For this review, take the finished solid that the model builds, in its own axes (mm). A direction names the side the tool comes from. Round coordinates to 2 decimals unless told otherwise and drop trailing zeros. Write each loop counter-clockwise with the first axis right and the second up, starting at its lowest first coordinate (ties: lowest second). Pieces come first, ordered by that corner, then holes. Notation, with made-up numbers: M 14,-7 L 54,-7 A24 cw 54,31 Z; hole C -28.75,-26.75 d2. An arc over 180 degrees is marked long. One line per question, with ' | ' between items.
```python
from build123d import *

# Parameters (mm, degrees)
BOSS_EXTRUDE1_DEPTH = 50.8
CUT_EXTRUDE2_REACH  = 8.35
SKETCH4_R           = 2.54
CUT_EXTRUDE1_REACH  = 8.35
SKETCH3_R           = 2.54
SKETCH3_R_2         = 14.224
CUT_EXTRUDE3_DEPTH  = 3.81


with BuildPart() as part:
    # Sketch2 → Boss-Extrude1 (new body)
    with BuildSketch(Plane(origin=(0, 0, 0), x_dir=(1, 0, 0), z_dir=(0, 1, 0))):
        Polygon((0, 58.372586566), (0, 0), (48.980415858, 0), (43.6521332, 6.35), (6.35, 6.35), (6.35, 50.804951253), align=None)
    extrude(amount=BOSS_EXTRUDE1_DEPTH)

    # Sketch4 → Cut-Extrude2 (cut, up to next)
    with BuildSketch(Plane(origin=(0, 0, -6.35), x_dir=(-1, 0, 0), z_dir=(0, 0, -1)), mode=Mode.PRIVATE) as cut_extrude2_sk1:
        with Locations((-37.7010666, 36.83)):
            Circle(SKETCH4_R)
    cut_extrude2_tool1 = extrude(cut_extrude2_sk1.sketch, amount=-CUT_EXTRUDE2_REACH, mode=Mode.PRIVATE) & part.part
    add(cut_extrude2_tool1.solids().sort_by_distance((37.701067, 36.83, -6.35))[0], mode=Mode.SUBTRACT)
    # Sketch4 → Cut-Extrude2 (cut, up to next)
    with BuildSketch(Plane(origin=(0, 0, -6.35), x_dir=(-1, 0, 0), z_dir=(0, 0, -1)), mode=Mode.PRIVATE) as cut_extrude2_sk2:
        with Locations((-12.3010666, 36.83)):
            Circle(SKETCH4_R)
    cut_extrude2_tool2 = extrude(cut_extrude2_sk2.sketch, amount=-CUT_EXTRUDE2_REACH, mode=Mode.PRIVATE) & part.part
    add(cut_extrude2_tool2.solids().sort_by_distance((12.301067, 36.83, -6.35))[0], mode=Mode.SUBTRACT)
    # Sketch4 → Cut-Extrude2 (cut, up to next)
    with BuildSketch(Plane(origin=(0, 0, -6.35), x_dir=(-1, 0, 0), z_dir=(0, 0, -1)), mode=Mode.PRIVATE) as cut_extrude2_sk3:
        with Locations((-37.7010666, 11.43)):
            Circle(SKETCH4_R)
    cut_extrude2_tool3 = extrude(cut_extrude2_sk3.sketch, amount=-CUT_EXTRUDE2_REACH, mode=Mode.PRIVATE) & part.part
    add(cut_extrude2_tool3.solids().sort_by_distance((37.701067, 11.43, -6.35))[0], mode=Mode.SUBTRACT)
    # Sketch4 → Cut-Extrude2 (cut, up to next)
    with BuildSketch(Plane(origin=(0, 0, -6.35), x_dir=(-1, 0, 0), z_dir=(0, 0, -1)), mode=Mode.PRIVATE) as cut_extrude2_sk4:
        with Locations((-12.3010666, 11.43)):
            Circle(SKETCH4_R)
    cut_extrude2_tool4 = extrude(cut_extrude2_sk4.sketch, amount=-CUT_EXTRUDE2_REACH, mode=Mode.PRIVATE) & part.part
    add(cut_extrude2_tool4.solids().sort_by_distance((12.301067, 11.43, -6.35))[0], mode=Mode.SUBTRACT)

    # Sketch3 → Cut-Extrude1 (cut, up to next)
    with BuildSketch(Plane(origin=(6.35, 0, 0), x_dir=(0, 0, -1), z_dir=(1, 0, 0)), mode=Mode.PRIVATE) as cut_extrude1_sk1:
        with Locations((13.335, 15.2019)):
            Circle(SKETCH3_R)
    cut_extrude1_tool1 = extrude(cut_extrude1_sk1.sketch, amount=-CUT_EXTRUDE1_REACH, mode=Mode.PRIVATE) & part.part
    add(cut_extrude1_tool1.solids().sort_by_distance((6.35, 15.2019, -13.335))[0], mode=Mode.SUBTRACT)
    # Sketch3 → Cut-Extrude1 (cut, up to next)
    with BuildSketch(Plane(origin=(6.35, 0, 0), x_dir=(0, 0, -1), z_dir=(1, 0, 0)), mode=Mode.PRIVATE) as cut_extrude1_sk2:
        with Locations((21.209, 34.2519)):
            Circle(SKETCH3_R_2)
    cut_extrude1_tool2 = extrude(cut_extrude1_sk2.sketch, amount=-CUT_EXTRUDE1_REACH, mode=Mode.PRIVATE) & part.part
    add(cut_extrude1_tool2.solids().sort_by_distance((6.35, 34.2519, -21.209))[0], mode=Mode.SUBTRACT)
    # Sketch3 → Cut-Extrude1 (cut, up to next)
    with BuildSketch(Plane(origin=(6.35, 0, 0), x_dir=(0, 0, -1), z_dir=(1, 0, 0)), mode=Mode.PRIVATE) as cut_extrude1_sk3:
        with Locations((40.259, 15.2019)):
            Circle(SKETCH3_R)
    cut_extrude1_tool3 = extrude(cut_extrude1_sk3.sketch, amount=-CUT_EXTRUDE1_REACH, mode=Mode.PRIVATE) & part.part
    add(cut_extrude1_tool3.solids().sort_by_distance((6.35, 15.2019, -40.259))[0], mode=Mode.SUBTRACT)
    # Sketch3 → Cut-Extrude1 (cut, up to next)
    with BuildSketch(Plane(origin=(6.35, 0, 0), x_dir=(0, 0, -1), z_dir=(1, 0, 0)), mode=Mode.PRIVATE) as cut_extrude1_sk4:
        with Locations((40.259, 42.1259)):
            Circle(SKETCH3_R)
    cut_extrude1_tool4 = extrude(cut_extrude1_sk4.sketch, amount=-CUT_EXTRUDE1_REACH, mode=Mode.PRIVATE) & part.part
    add(cut_extrude1_tool4.solids().sort_by_distance((6.35, 42.1259, -40.259))[0], mode=Mode.SUBTRACT)

    # Sketch5 → Cut-Extrude3 (cut)
    with BuildSketch(Plane.XZ):
        Polygon((0, -48.643822138), (40.817013215, 0), (36.838131797, 0), (0, -43.901975914), align=None)
    extrude(amount=-CUT_EXTRUDE3_DEPTH, mode=Mode.SUBTRACT)


solid = part.part
```
Item 1: Take a section at D-D (x = 13). Write out the cut boundary in (y, z).
Results:
outline: M 0,-6.35 L 8.99,-6.35 L 8.99,0 L 0,0 Z; M 13.87,-6.35 L 34.39,-6.35 L 34.39,0 L 13.87,0 Z; M 39.27,-6.35 L 50.8,-6.35 L 50.8,0 L 39.27,0 Z
Item 2: Take a section at C-C (y = 46). Write out the cut boundary in (x, z).
Results:
outline: M 0,-58.37 L 6.35,-50.8 L 6.35,-29.23 L 0,-29.23 Z; M 0,-13.19 L 6.35,-13.19 L 6.35,-6.35 L 43.65,-6.35 L 48.98,0 L 0,0 Z
Item 3: Mouldability with a two-part tool opening along Y and no side actions: class faces 1 (the face through (36, 3.81, -3)), 2 (the face through (14.317, 9.884, -3.219)), 3 (the face through (0, 19, -30)) as +Y half, -Y half, draft (parallel to the pull), parting line (faces both ways), or undercut.
Results:
face 1: -Y half | face 2: undercut | face 3: draft
Item 4: Take a section at B-B (z = -30). Write out the cut boundary in (x, y).
Results:
outline: M 0,0 L 6.35,0 L 6.35,23.07 L 0,23.07 Z; M 0,45.43 L 6.35,45.43 L 6.35,50.8 L 0,50.8 Z
Item 5: Take a section at A-A (y = 11.43). Write out the cut boundary in (x, z).
Results:
outline: M 0,-58.37 L 6.35,-50.8 L 6.35,-6.35 L 9.76,-6.35 L 9.76,0 L 0,0 Z; M 14.84,-6.35 L 35.16,-6.35 L 35.16,0 L 14.84,0 Z; M 40.24,-6.35 L 43.65,-6.35 L 48.98,0 L 40.24,0 Z
Item 6: Machinability: for faces 4 (the face through (25, 25, -6.35)), 5 (the face through (34.21, 1.88, -3.13)), 6 (the face through (3.22, 15.31, -37.72)), which of the approach directions +Z, -Z, +X, -X, +Y, -Y give a long, thin tool a straight path to every point of the face, cutting with its end or side? Answer none if there is none.
Results:
face 4: -Z, +X, +Y, -Y | face 5: -Y | face 6: +X, -X
Item 7: To check wall thickness, follow line 1 along X through (y, z) = (36, -4); line 2 along Y through (x, z) = (4, -41.5); line 3 along Z through (x, y) = (19, 33.5). State the ranges of each line that lie inside material, in increasing order. Write a range as from..to.
Results:
line 1: 0..9.9, 14.7..35.3, 40.1..45.62 | line 2: 3.81..12.99, 17.42..39.91, 44.34..50.8 | line 3: -6.35..0
Item 8: Insertion check: pin 1 Ø6 at (x, y) = (37.7, 36.83) entering from -Z; pin 2 Ø1 at (y, z) = (44, -49.5) entering from +X; pin 3 Ø2 at (x, y) = (35.5, 5.5) entering from -Z. Each pin has a flat end and moves straight along its axis. Give the tip position at first contact, or say it passes through.
Results:
pin 1: z = -6.35 | pin 2: x = 6.35 | pin 3: z = -6.35
